from build123d import *

# Parameters (mm, degrees)
F0_W         = 25
F0_H         = 15.1
F1_DEPTH     = 7.5
F2_W         = 12.2
F2_H         = 4.6
F3_DEPTH     = 9.95
F4_W         = 3.9
F4_H         = 8.9
F5_DEPTH     = 25
F6_SIZE      = 1
F7_C1_SIZE   = 1
F7_C2_SIZE   = 1
F7_C3_SIZE   = 1
F7_C4_SIZE   = 1
F7_C5_SIZE   = 1
F7_C6_SIZE   = 1
F7_C7_SIZE   = 1
F7_C8_SIZE   = 1
F8_R         = 20.5
F9_DEPTH     = 25
F10_T2_ANGLE = 49.7995158882
F10_T4_ANGLE = 49.7995158882
F10_T6_ANGLE = 49.7995158882
F10_T8_ANGLE = 49.7995158882
F12_DEPTH    = 25
F13_SIZE     = 1
F14_W        = 6.9057337241
F14_H        = 9.9417776801
F15_DEPTH    = 0.5


# Not quite as in the source:
# - a fillet or chamfer that OpenCascade refuses, or shapes differently, is made with other operations: its cross-section is extruded or revolved along the edge and cut away or added


with BuildPart() as f1:
    # F0 (on Top) → F1 (new body)
    with BuildSketch(Plane.XY):
        with Locations((12.5, 0)):
            Rectangle(F0_W, F0_H)
    extrude(amount=F1_DEPTH)

    # F2 (on face) → F3 (cut)
    with BuildSketch(Plane(origin=(0, 0, 0), x_dir=(0, -1, 0), z_dir=(-1, 0, 0))):
        with Locations((0, 3.75)):
            Rectangle(F2_W, F2_H)
    extrude(amount=-F3_DEPTH, mode=Mode.SUBTRACT)

    # F4 (on face) → F5 (cut)
    with BuildSketch(Plane.XY.offset(7.5)):
        with Locations((3.9, 0)):
            Rectangle(F4_W, F4_H)
    extrude(amount=-F5_DEPTH, mode=Mode.SUBTRACT)

    # F6
    f6_edges = [f1.edges().sort_by_distance(p)[0] for p in [
        (25, -7.55, 3.75),
        (25, 7.55, 3.75),
        (25, 0, 0),
        (25, 0, 7.5),
    ]]
    chamfer(f6_edges, length=F6_SIZE)

    # F7: chamfer of 1 on 8 edges, made by hand

    # F7_c1
    f7_c1_edges = [f1.edges().sort_by_distance(p)[0] for p in [
        (12, -7.55, 0),
    ]]
    chamfer(f7_c1_edges, length=F7_C1_SIZE)

    # F7_c2
    f7_c2_edges = [f1.edges().sort_by_distance(p)[0] for p in [
        (0, -7.55, 4.25),
    ]]
    chamfer(f7_c2_edges, length=F7_C2_SIZE)

    # F7_c3
    f7_c3_edges = [f1.edges().sort_by_distance(p)[0] for p in [
        (12.5, -7.55, 7.5),
    ]]
    chamfer(f7_c3_edges, length=F7_C3_SIZE)

    # F7_c4
    f7_c4_edges = [f1.edges().sort_by_distance(p)[0] for p in [
        (0, 0.5, 0),
    ]]
    chamfer(f7_c4_edges, length=F7_C4_SIZE)

    # F7_c5
    f7_c5_edges = [f1.edges().sort_by_distance(p)[0] for p in [
        (12.5, 7.55, 0),
    ]]
    chamfer(f7_c5_edges, length=F7_C5_SIZE)

    # F7_c6
    f7_c6_edges = [f1.edges().sort_by_distance(p)[0] for p in [
        (0, 0.5, 7.5),
    ]]
    chamfer(f7_c6_edges, length=F7_C6_SIZE)

    # F7_c7
    f7_c7_edges = [f1.edges().sort_by_distance(p)[0] for p in [
        (12.5, 7.55, 7.5),
    ]]
    chamfer(f7_c7_edges, length=F7_C7_SIZE)

    # F7_c8
    f7_c8_edges = [f1.edges().sort_by_distance(p)[0] for p in [
        (0, 7.55, 3.75),
    ]]
    chamfer(f7_c8_edges, length=F7_C8_SIZE)

    # F8 (on face) → F9 (cut)
    with BuildSketch(Plane.XY.offset(7.5)):
        with Locations((16.8532188982, 26.55)):
            Circle(F8_R)
        with Locations((16.8532188982, -26.55)):
            Circle(F8_R)
    extrude(amount=-F9_DEPTH, mode=Mode.SUBTRACT)

    # F10: chamfer of 1 on 4 edges, made by hand

    # F10_s1 → F10_t2 (revolve, cut)
    with BuildSketch(Plane(origin=(24.005003563, -11.1426284002, 0), x_dir=(0, 0, 1), z_dir=(0.907045793, -0.4210319814, 0))):
        Polygon((7.5, -4.5136783409), (6.5, -3.5136783409), (7.5, -3.5136783409), align=None)
    revolve(axis=Axis((16.8532188982, -26.55, 7.5), (0, 0, 1)), revolution_arc=F10_T2_ANGLE, mode=Mode.SUBTRACT)

    # F10_s3 → F10_t4 (revolve, cut)
    with BuildSketch(Plane(origin=(3.7263637991, -1.7297013511, 0), x_dir=(0, 0, 1), z_dir=(-0.907045793, 0.4210319814, 0))):
        Polygon((7.5, 9.6778099504), (6.5, 10.6778099504), (7.5, 10.6778099504), align=None)
    revolve(axis=Axis((16.8532188982, 26.55, 7.5), (0, 0, 1)), revolution_arc=F10_T4_ANGLE, mode=Mode.SUBTRACT)

    # F10_s5 → F10_t6 (revolve, cut)
    with BuildSketch(Plane(origin=(24.005003563, -11.1426284002, 0), x_dir=(0, 0, 1), z_dir=(0.907045793, -0.4210319814, 0))):
        Polygon((1, -3.5136783409), (0, -4.5136783409), (0, -3.5136783409), align=None)
    revolve(axis=Axis((16.8532188982, -26.55, 0), (0, 0, 1)), revolution_arc=F10_T6_ANGLE, mode=Mode.SUBTRACT)

    # F10_s7 → F10_t8 (revolve, cut)
    with BuildSketch(Plane(origin=(3.7263637991, -1.7297013511, 0), x_dir=(0, 0, 1), z_dir=(-0.907045793, 0.4210319814, 0))):
        Polygon((1, 10.6778099504), (0, 9.6778099504), (0, 10.6778099504), align=None)
    revolve(axis=Axis((16.8532188982, 26.55, 0), (0, 0, 1)), revolution_arc=F10_T8_ANGLE, mode=Mode.SUBTRACT)

    # F11 (on face) → F12 (cut)
    with BuildSketch(Plane.XY.offset(7.5)):
        with BuildLine():
            ThreePointArc((11.1193139957, -4.2761962258), (16.8082592809, -3.5500439428), (22.5, -4.2539496056))
            Line((22.5, -4.2539496056), (22.5, 4.2539496056))
            ThreePointArc((22.5, 4.2539496056), (16.8082592809, 3.5500439428), (11.1193139957, 4.2761962258))
            Line((11.1193139957, 4.2761962258), (11.1193139957, -4.2761962258))
        make_face()
    extrude(amount=-F12_DEPTH, mode=Mode.SUBTRACT)

    # F13
    f13_edges = [f1.edges().sort_by_distance(p)[0] for p in [
        (11.119314, 0, 7.5),
        (16.808259, 3.550044, 7.5),
        (22.5, 0, 7.5),
        (16.808259, -3.550044, 7.5),
        (11.119314, 0, 0),
        (16.808259, 3.550044, 0),
        (22.5, 0, 0),
        (16.808259, -3.550044, 0),
    ]]
    chamfer(f13_edges, length=F13_SIZE)

    # F14 (on face) → F15 (join)
    with BuildSketch(Plane(origin=(0, 0, 0), x_dir=(1, 0, 0), z_dir=(0, 0, -1))):
        with Locations((4.9177300534, -0.0320777763)):
            Rectangle(F14_W, F14_H)
    extrude(amount=-F15_DEPTH)


solid = f1.part
Could you check a few things on this model? Use its own coordinates, in mm. A direction names the side the tool comes from. Round coordinates to 2 decimals unless told otherwise and drop trailing zeros. Write each loop counter-clockwise with the first axis right and the second up, starting at its lowest first coordinate (ties: lowest second). Pieces come first, ordered by that corner, then holes. Notation, with made-up numbers: (70, 66.25) -> (124, 66.25) arc R24 cw to (124, 90.25) -> close; hole circle Ø11 at (10, 40). An arc over 180 degrees is marked (long way). Use a Markdown table: item, result.
1. If we section it at C-C (x = 6.75): List the corners of the cut face in (y, z) for me, then the cut area to 3 significant figures.
Answer key:
| item | result |
|---|---|
| outline | (-7.55, 1) -> (-6.55, 0) -> (6.55, 0) -> (7.55, 1) -> (7.55, 6.5) -> (6.55, 7.5) -> (-6.55, 7.5) -> (-7.55, 6.5) -> close; hole (-6.1, 1.45) -> (6.1, 1.45) -> (6.1, 6.05) -> (-6.1, 6.05) -> close |
| area | 55.1 mm^2 |
2. If we section it at D-D (x = 4.25): List the corners of the cut face in (y, z) for me, then the cut area to 3 significant figures.
Answer key:
| item | result |
|---|---|
| outline | (-7.55, 1) -> (-6.55, 0) -> (6.55, 0) -> (7.55, 1) -> (7.55, 6.5) -> (6.55, 7.5) -> (4.45, 7.5) -> (4.45, 6.05) -> (6.1, 6.05) -> (6.1, 1.45) -> (4.45, 1.45) -> (4.45, 0.5) -> (-4.45, 0.5) -> (-4.45, 1.45) -> (-6.1, 1.45) -> (-6.1, 6.05) -> (-4.45, 6.05) -> (-4.45, 7.5) -> (-6.55, 7.5) -> (-7.55, 6.5) -> close |
| area | 33.8 mm^2 |
3. If we section it at A-A (y = -0.25): List the corners of the cut face in (x, z) for me.
Answer key:
| item | result |
|---|---|
| outline | (0, 1) -> (1, 0) -> (10.12, 0) -> (11.12, 1) -> (11.12, 6.5) -> (10.12, 7.5) -> (5.85, 7.5) -> (5.85, 6.05) -> (9.95, 6.05) -> (9.95, 1.45) -> (5.85, 1.45) -> (5.85, 0.5) -> (1.95, 0.5) -> (1.95, 1.45) -> (0, 1.45) -> close; (0, 6.05) -> (1.95, 6.05) -> (1.95, 7.5) -> (1, 7.5) -> (0, 6.5) -> close; (22.5, 1) -> (23.5, 0) -> (24, 0) -> (25, 1) -> (25, 6.5) -> (24, 7.5) -> (23.5, 7.5) -> (22.5, 6.5) -> close |
4. If we section it at B-B (z = 1.75): List the corners of the cut face in (x, y) for me, then the cut area to 3 significant figures.
Answer key:
| item | result |
|---|---|
| outline | (0, -6.55) -> (1, -7.55) -> (9.16, -7.55) arc R20.5 cw to (24.16, -7.39) -> (25, -6.55) -> (25, 6.55) -> (24.16, 7.39) arc R20.5 cw to (9.16, 7.55) -> (1, 7.55) -> (0, 6.55) -> (0, 6.1) -> (9.95, 6.1) -> (9.95, -6.1) -> (0, -6.1) -> close; hole (11.12, -4.28) arc R23 cw to (22.5, -4.25) -> (22.5, 4.25) arc R23 cw to (11.12, 4.28) -> close |
| area | 137 mm^2 |
5. We'd pull the mould along Y, two halves only. Please class faces 5 (the face through (4, 4.45, 7)), 6 (the face through (0.51, 7.06, 3.7)), 7 (the face through (0, -0.5, 6.2)), 8 (the face through (16.85, -5.77, 0.72)): +Y half, -Y half, draft (parallel to the pull), parting line (faces both ways), or undercut.
Answer key:
| item | result |
|---|---|
| face 5 | undercut |
| face 6 | +Y half |
| face 7 | draft |
| face 8 | -Y half |
6. For pin 1 Ø1 at (x, z) = (10, 1.5) entering from -Y; pin 2 Ø1.2 at (x, y) = (3.5, -2) entering from +Z; pin 3 Ø1 at (x, z) = (17.5, 5.5) entering from -Y, each with a flat end and sliding along its axis, tell me the tip position at first contact or that it passes through.
Answer key:
| item | result |
|---|---|
| pin 1 | stops at y = -7.41 |
| pin 2 | stops at z = 0.5 |
| pin 3 | stops at y = -6.08 |
7. Which directions (+Z, -Z, +X, -X, +Y, -Y) give clear straight access to the entire face, cutting with the end or side of a thin tool? Please do faces 1 (the face through (23, -0.1, 0.5)), 2 (the face through (23, 0, 7)), 3 (the face through (9.95, 0, 4)), 4 (the face through (0.5, -0.1, 0.5)).
Answer key:
| item | result |
|---|---|
| face 1 | -Z |
| face 2 | +Z |
| face 3 | -X |
| face 4 | -Z, -X, +Y, -Y |
8. Please list where these lines run through material, in increasing order: probe 1 along Y at (x, z) = (7.75, 2.5); probe 2 along X at (y, z) = (-1.5, 3.25); probe 3 along Z at (x, y) = (6.5, -2.5).
Answer key:
| item | result |
|---|---|
| probe 1 | y = -7.55 to -6.1, 6.1 to 7.55 |
| probe 2 | x = 9.95 to 11.12, 22.5 to 25 |
| probe 3 | z = 0 to 1.45, 6.05 to 7.5 |
